Design review of the part built by this model. Coordinates are the model's own, in mm. Face numbers are marked on the shaded views. Give positions to 0.01 mm unless a question says otherwise; leave off trailing zeros. Write each loop counter-clockwise with the first axis right and the second up, starting at its lowest first coordinate (ties: lowest second). Pieces come first, ordered by that corner, then holes. Notation, with made-up numbers: M 54.25,44.25 L 100.25,44.25 A14 cw 100.25,66.25 Z; hole C 2,23 d2. An arc over 180 degrees is marked long. Answer in a Markdown table with one row per item.
```python
from build123d import *

# Parameters (mm, degrees)
SKETCH1_W           = 75
SKETCH1_H           = 9.5
BOSS_EXTRUDE1_DEPTH = 6
SKETCH2_R           = 1
SKETCH2_W           = 63
SKETCH2_H           = 2
CUT_EXTRUDE1_DEPTH  = 3


with BuildPart() as part:
    # Sketch1 → Boss-Extrude1 (new body)
    with BuildSketch(Plane(origin=(0, 0, 0), x_dir=(1, 0, 0), z_dir=(0, 1, 0))):
        with Locations((37.5, 4.75)):
            Rectangle(SKETCH1_W, SKETCH1_H)
    extrude(amount=BOSS_EXTRUDE1_DEPTH)

    # Sketch2 → Cut-Extrude1 (cut)
    with BuildSketch(Plane(origin=(0, 6, 0), x_dir=(1, 0, 0), z_dir=(0, 1, 0))):
        with Locations((2.5, 4.75)):
            Circle(SKETCH2_R)
        with Locations((72.5, 4.75)):
            Circle(SKETCH2_R)
        with Locations((37.5, 4.75)):
            Rectangle(SKETCH2_W, SKETCH2_H)
    extrude(amount=-CUT_EXTRUDE1_DEPTH, mode=Mode.SUBTRACT)


solid = part.part
```
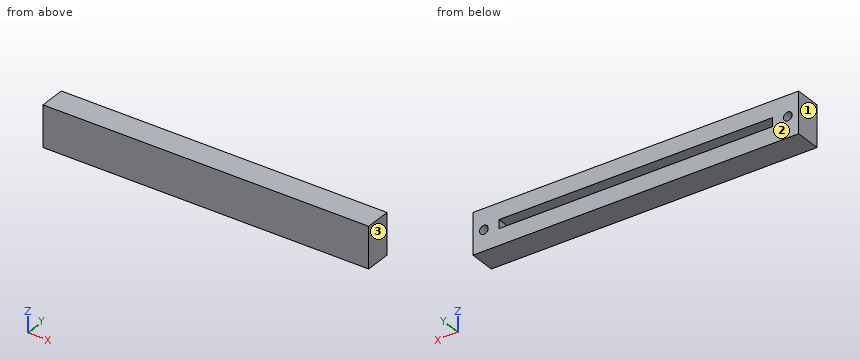
1) The part is to be moulded in two halves that separate along X. For the marked faces 1, 2 and 3, say which applies: released by +X, released by -X, zero draft, split by the parting line, or undercut.
Geometry says:
| item | result |
|---|---|
| face 1 | released by -X |
| face 2 | zero draft |
| face 3 | released by +X |
2) Insertion check: P1, Ø0.6, axis at x = 73, z = -5, coming from the +Y side. The pin has a flat end and moves straight along its axis. Give the tip position at first contact, or say it passes through.
Geometry says:
| item | result |
|---|---|
| P1 | y = 3 |
3) Add section A-A (y = 3.7). Write out the cut boundary in (x, z), and give its area (3 significant figures).
Geometry says:
| item | result |
|---|---|
| outline | M 0,-9.5 L 75,-9.5 L 75,0 L 0,0 Z; hole C 2.5,-4.75 d2; hole M 6,-5.75 L 69,-5.75 L 69,-3.75 L 6,-3.75 Z; hole C 72.5,-4.75 d2 |
| area | 580 mm^2 |
4) To check wall thickness, follow probe 1 along X at (y, z) = (5.35, -4.75); probe 2 along Z at (x, y) = (47, 3.75); probe 3 along X at (y, z) = (5.55, -4). State the ranges of each line that lie inside material, in increasing order. Write a range as [from, to].
Geometry says:
| item | result |
|---|---|
| probe 1 | [0, 1.5], [3.5, 6], [69, 71.5], [73.5, 75] |
| probe 2 | [-9.5, -5.75], [-3.75, 0] |
| probe 3 | [0, 1.84], [3.16, 6], [69, 71.84], [73.16, 75] |
5) Add section B-B (x = 72.5). Write out the cut boundary in (y, z).
Geometry says:
| item | result |
|---|---|
| outline | M 0,-9.5 L 6,-9.5 L 6,-5.75 L 3,-5.75 L 3,-3.75 L 6,-3.75 L 6,0 L 0,0 Z |
